Could you check a few things on this model? Use its own coordinates, in mm. Face numbers are marked on the shaded views. Give positions to 0.01 mm unless a question says otherwise; leave off trailing zeros. Order: outer loops, then holes, each group sorted by start corner. A loop starts at its lowest first (then second) coordinate and runs counter-clockwise, first axis right, second up. Notation, with made-up numbers: (-32.75, -27.5) - (15.25, -27.5) arc R14 cw to (15.25, -19.5) - close; hole circle Ø6 at (-7, 24.25). An arc over 180 degrees is marked (long way). Put each result on its own line as item: value.
from build123d import *

# Parameters (mm, degrees)
SKETCH1_R           = 1.27
SKETCH1_R_2         = 0.635
BOSS_EXTRUDE1_DEPTH = 1.651
SKETCH2_W           = 1.27
SKETCH2_H           = 2.032
BOSS_EXTRUDE2_DEPTH = 1.3208


with BuildPart() as part:
    # Sketch1 → Boss-Extrude1 (new body)
    with BuildSketch(Plane(origin=(0, 0, 0), x_dir=(1, 0, 0), z_dir=(0, 1, 0))):
        with BuildLine():
            Line((2.032, 0), (17.399, 0))
            ThreePointArc((17.399, 0), (18.835840979, 0.595159021), (19.431, 2.032))
            Line((19.431, 2.032), (19.431, 15.748))
            ThreePointArc((19.431, 15.748), (18.835840979, 17.184840979), (17.399, 17.78))
            Line((17.399, 17.78), (2.032, 17.78))
            ThreePointArc((2.032, 17.78), (0.595159021, 17.184840979), (0, 15.748))
            Line((0, 15.748), (0, 2.032))
            ThreePointArc((0, 2.032), (0.595159021, 0.595159021), (2.032, 0))
        make_face()
        with Locations((2.54, 15.24)):
            Circle(SKETCH1_R, mode=Mode.SUBTRACT)
        with Locations((16.891, 15.24)):
            Circle(SKETCH1_R, mode=Mode.SUBTRACT)
        with Locations((2.0955, 2.413)):
            Circle(SKETCH1_R_2, mode=Mode.SUBTRACT)
        with Locations((4.6355, 2.413)):
            Circle(SKETCH1_R_2, mode=Mode.SUBTRACT)
        with Locations((7.1755, 2.413)):
            Circle(SKETCH1_R_2, mode=Mode.SUBTRACT)
        with Locations((9.7155, 2.413)):
            Circle(SKETCH1_R_2, mode=Mode.SUBTRACT)
        with Locations((12.2555, 2.413)):
            Circle(SKETCH1_R_2, mode=Mode.SUBTRACT)
        with Locations((14.7955, 2.413)):
            Circle(SKETCH1_R_2, mode=Mode.SUBTRACT)
        with Locations((17.3355, 2.413)):
            Circle(SKETCH1_R_2, mode=Mode.SUBTRACT)
    extrude(amount=BOSS_EXTRUDE1_DEPTH)

    # Sketch2 → Boss-Extrude2 (add)
    with BuildSketch(Plane(origin=(0, 1.651, 0), x_dir=(1, 0, 0), z_dir=(0, 1, 0))):
        with Locations((9.0805, 7.874)):
            Rectangle(SKETCH2_W, SKETCH2_H)
        Polygon((8.4455, 8.89), (9.7155, 8.89), (9.7155, 6.858), (10.9855, 6.858), (10.9855, 10.922), (8.4455, 10.922), align=None)
    extrude(amount=BOSS_EXTRUDE2_DEPTH)


solid = part.part
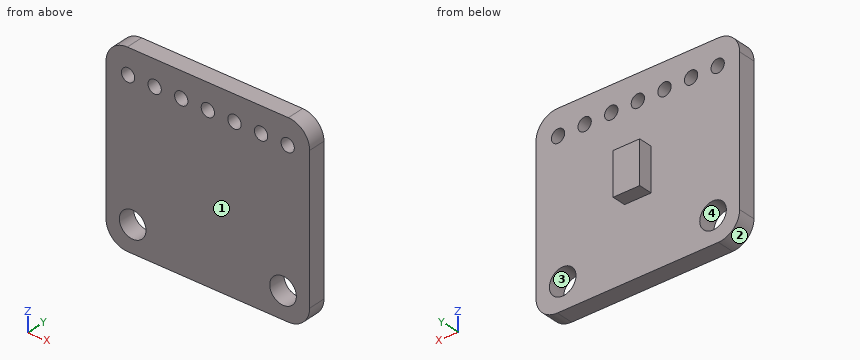
1) Suppose I cut it at B-B, the plane x = 16. List the corners of the cut face in (y, z) for me (3 decimals), and give its area (3 significant figures).
Filled in:
outline: (0, -17.78) - (1.651, -17.78) - (1.651, -16.145) - (0, -16.145) - close; (0, -14.335) - (1.651, -14.335) - (1.651, 0) - (0, 0) - close
area: 26.4 mm^2
2) Suppose I cut it at A-A, the plane z = -15.24. List the corners of the cut face in (x, y) for me, and give its area (3 significant figures).
Filled in:
outline: (0, 0) - (1.27, 0) - (1.27, 1.65) - (0, 1.65) - close; (3.81, 0) - (15.62, 0) - (15.62, 1.65) - (3.81, 1.65) - close; (18.16, 0) - (19.43, 0) - (19.43, 1.65) - (18.16, 1.65) - close
area: 23.7 mm^2
3) If I drill on line 1 (X direction, y = 1.1, z = -15.24); line 2 (X direction, y = 1.05, z = -16); line 3 (Y direction, x = 12.5, z = -13), over which ranges is the centre line in solid material (lowest first)? Write a range as [from, to].
Filled in:
line 1: x = [0, 1.27], [3.81, 15.62], [18.16, 19.43]
line 2: x = [0.02, 1.52], [3.56, 15.87], [17.91, 19.42]
line 3: y = [0, 1.65]
4) I'm going to push a flat-ended pin straight in: pin 1 (4 mm diameter, centred on x = 16.891, z = -15.24, fed in from +Y). Where does the tip first touch, or does it pass through?
Filled in:
pin 1: stops at y = 1.65
5) We'd pull the mould along X, two halves only. Please class the marked faces 1, 2, 3 and 4: pulls with the +X half, pulls with the -X half, needs draft (parallel to the pull), parting line crosses it, or undercut.
Filled in:
face 1: needs draft
face 2: pulls with the -X half
face 3: undercut
face 4: undercut
6) Suppose I cut it at C-C, the plane z = -10. List the corners of the cut face in (x, y) for me, and give its area (3 significant figures).
Filled in:
outline: (0, 0) - (19.43, 0) - (19.43, 1.65) - (10.99, 1.65) - (10.99, 2.97) - (8.45, 2.97) - (8.45, 1.65) - (0, 1.65) - close
area: 35.4 mm^2
7) Suppose I cut it at D-D, the plane y = 1.2. State how many separate pieces and enclosed holes the cut face has, and give its area (3 significant figures).
Filled in:
separate pieces: 1
enclosed holes: 9
area: 323 mm^2
